from build123d import *

# Parameters (mm, degrees)
SKETCH1_W           = 40
SKETCH1_H           = 6.35
BOSS_EXTRUDE1_DEPTH = 34.925
SKETCH2_R           = 1.651
CUT_EXTRUDE1_DEPTH  = 8
SKETCH3_R           = 10
CUT_EXTRUDE2_DEPTH  = 54.479698251
SKETCH4_R           = 1.65
CUT_EXTRUDE3_DEPTH  = 54.479698328
CIRPATTERN1_COUNT   = 6


with BuildPart() as part:
    # Sketch1 → Boss-Extrude1 (new body)
    with BuildSketch(Plane.XY):
        with Locations((20, 3.175)):
            Rectangle(SKETCH1_W, SKETCH1_H)
    extrude(amount=BOSS_EXTRUDE1_DEPTH)

    # Sketch2 → Cut-Extrude1 (cut)
    with BuildSketch(Plane.XY.offset(34.925)):
        with Locations((15.174, 3.472079932)):
            Circle(SKETCH2_R)
        with Locations((24.826, 3.472079932)):
            Circle(SKETCH2_R)
    cut_extrude1 = extrude(amount=-CUT_EXTRUDE1_DEPTH, mode=Mode.SUBTRACT)

    # Mirror1: Cut-Extrude1 across plane
    add(cut_extrude1.mirror(Plane.XY.offset(17.4625)), mode=Mode.SUBTRACT)

    # Sketch3 → Cut-Extrude2 (cut, through all)
    with BuildSketch(Plane(origin=(0, 6.35, 0), x_dir=(1, 0, 0), z_dir=(0, 1, 0))):
        with Locations(Location((20, -17.4625, 0), (0, 0, 270))):
            Circle(SKETCH3_R)
    extrude(amount=-CUT_EXTRUDE2_DEPTH, mode=Mode.SUBTRACT)

    # Sketch4 → Cut-Extrude3 (cut, through all)
    with BuildSketch(Plane(origin=(0, 6.35, 0), x_dir=(1, 0, 0), z_dir=(0, 1, 0))):
        with Locations(Location((20, -1.9625, 0), (0, 0, 270))):
            Circle(SKETCH4_R)
    cut_extrude3 = extrude(amount=-CUT_EXTRUDE3_DEPTH, mode=Mode.SUBTRACT)

    # CirPattern1: Cut-Extrude3 ×6 about axis
    cirpattern1_axis = Axis((20, 0, 17.4625), (0, 1, 0))
    for i in range(1, CIRPATTERN1_COUNT):
        add(cut_extrude3.rotate(cirpattern1_axis, i * 360 / CIRPATTERN1_COUNT), mode=Mode.SUBTRACT)


solid = part.part
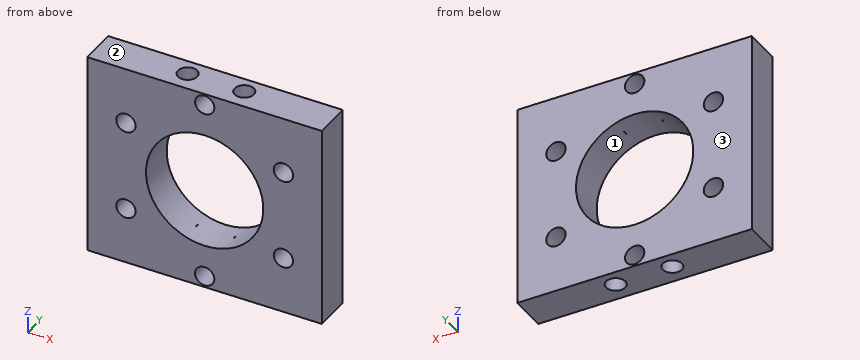
Input: part model. Units: mm. Frame: model coordinates. Face numbers are marked on the shaded views. Give positions to 0.01 mm unless a question says otherwise; leave off trailing zeros. Loops run counter-clockwise (first coordinate to the right, second up) from the corner with the lowest first, then second, coordinate; pieces in that order, holes last. Notation, with made-up numbers: (8.25, 1) -> (58.25, 1) arc R7 ccw to (58.25, 9) -> close; hole circle Ø2 at (36.25, 40). An arc over 180 degrees is marked (long way). Answer as a JSON object with one key per item and string values. Group by question number.
Item 1: Line query: probe 1 along X at (y, z) = (2.5, 5.5); probe 2 along Z at (x, y) = (5.5, 4) (3 decimals); probe 3 along X at (y, z) = (2, 31). Output: solid intervals per line, ascending.
Item 2: Cut plane A-A, the plane x = 20. State how many separate pieces and enclosed holes the cut face has, and give its area (3 significant figures).
Item 3: Cut plane B-B, the plane z = 18.5. Return the cut outline in (x, y), and give its area (3 significant figures).
Item 4: Pin query (flat end, axial travel): P1, Ø1, axis at x = 15.5, y = 4, coming from the -Z side; P2, Ø1, axis at x = 24, y = 3.5, coming from the +Z side (3 decimals). Return the tip coordinate at first contact, or that it passes through.
Item 5: Pull-direction query (Z, two-part tool) for the marked faces 1, 2 and 3; classes: released by +Z, released by -Z, zero draft, split by the parting line, or undercut.
Item 6: Cut plane D-D, the plane x = 33. Return the cut outline in (y, z) (3 decimals).
Checks:
{
 "1": {"probe 1": "x = 0 to 13.84, 16.51 to 23.49, 26.16 to 40", "probe 2": "z = 0 to 8.462, 10.963 to 23.962, 26.463 to 34.925", "probe 3": "x = 0 to 14.43, 15.92 to 24.08, 25.57 to 40"},
 "2": {"separate pieces": "4", "enclosed holes": "0", "area": "52.9 mm²"},
 "3": {"outline": "(0, 0) -> (10.05, 0) -> (10.05, 6.35) -> (0, 6.35) -> close; (29.95, 0) -> (40, 0) -> (40, 6.35) -> (29.95, 6.35) -> close", "area": "128 mm²"},
 "4": {"P1": "stops at z = 8", "P2": "stops at z = 26.925"},
 "5": {"face 1": "undercut", "face 2": "released by +Z", "face 3": "zero draft"},
 "6": {"outline": "(0, 0) -> (6.35, 0) -> (6.35, 8.118) -> (0, 8.118) -> close; (0, 11.307) -> (6.35, 11.307) -> (6.35, 23.618) -> (0, 23.618) -> close; (0, 26.807) -> (6.35, 26.807) -> (6.35, 34.925) -> (0, 34.925) -> close"}
}
